The listing builds one solid part. Answer for the finished solid, in the listing's coordinates (mm). Face numbers are marked on the shaded views. A direction names the side the tool comes from. Coordinates: 2 decimals unless noted, no trailing zeros. Order: outer loops, then holes, each group sorted by start corner. A loop starts at its lowest first (then second) coordinate and runs counter-clockwise, first axis right, second up. Notation, with made-up numbers: (9.25, 53) -> (40.25, 53) arc R26 cw to (40.25, 85) -> close; hole circle Ø11 at (85, -34.5). An arc over 180 degrees is marked (long way). Return JSON: item names as keys, results as strings.
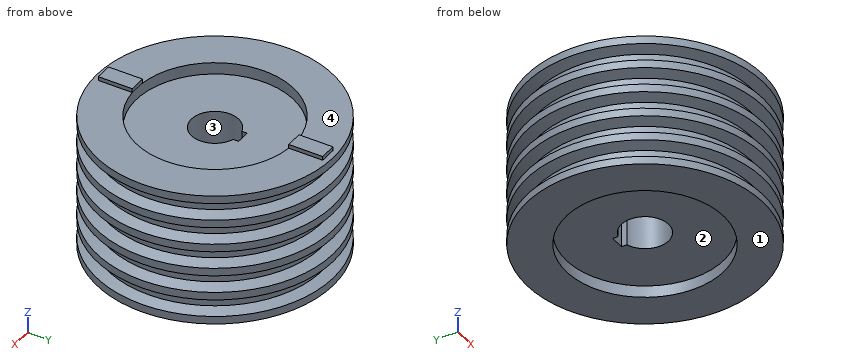
```python
from build123d import *

# Parameters (mm, degrees)
SKETCH1_R           = 150
BOSS_EXTRUDE1_DEPTH = 85
SKETCH3_R           = 30
CUT_EXTRUDE1_DEPTH  = 272.845544381
SKETCH4_R           = 100
SKETCH4_R_2         = 30
CUT_EXTRUDE2_DEPTH  = 15
SKETCH5_W           = 18
SKETCH5_H           = 11
CUT_EXTRUDE3_DEPTH  = 263.726093108
SKETCH10_W          = 21.256971554
SKETCH10_H          = 43.218095202
BOSS_EXTRUDE2_DEPTH = 5


with BuildPart() as part:
    # Sketch1 → Boss-Extrude1 (new, symmetric)
    with BuildSketch(Plane.XY):
        Circle(SKETCH1_R)
    extrude(amount=BOSS_EXTRUDE1_DEPTH, both=True)

    # Sketch3 → Cut-Extrude1 (cut, through all)
    with BuildSketch(Plane.XY.offset(85)):
        Circle(SKETCH3_R)
    extrude(amount=-CUT_EXTRUDE1_DEPTH, mode=Mode.SUBTRACT)

    # Sketch4 → Cut-Extrude2 (cut)
    with BuildSketch(Plane.XY.offset(85)):
        Circle(SKETCH4_R)
        Circle(SKETCH4_R_2, mode=Mode.SUBTRACT)
    cut_extrude2 = extrude(amount=-CUT_EXTRUDE2_DEPTH, mode=Mode.SUBTRACT)

    # Mirror1: Cut-Extrude2 across plane
    add(cut_extrude2.mirror(Plane.XY), mode=Mode.SUBTRACT)

    # Sketch5 → Cut-Extrude3 (cut, through all)
    with BuildSketch(Plane.XY.offset(70)):
        with Locations((0, 30)):
            Rectangle(SKETCH5_W, SKETCH5_H)
    extrude(amount=-CUT_EXTRUDE3_DEPTH, mode=Mode.SUBTRACT)

    # Sketch9 → Cut-Revolve2 (revolve, cut)
    with BuildSketch(Plane(origin=(0, 0, 0), x_dir=(1, 0, 0), z_dir=(0, 1, 0))):
        Polygon((150, 75), (136, 70.71977046), (136, 57.28022954), (150, 53), align=None)
        Polygon((150, 43), (150, 21), (136, 25.28022954), (136, 38.71977046), align=None)
        Polygon((150, 11), (136, 6.71977046), (136, -6.71977046), (150, -11), align=None)
        Polygon((150, -21), (150, -43), (136, -38.71977046), (136, -25.28022954), align=None)
        Polygon((150, -53), (136, -57.28022954), (136, -70.71977046), (150, -75), align=None)
    revolve(axis=Axis((0, 0, 0), (0, 0, -1)), mode=Mode.SUBTRACT)

    # Sketch10 → Boss-Extrude2 (add)
    with BuildSketch(Plane.XY.offset(85)):
        with Locations((-1.274543696, 121.17060528)):
            Rectangle(SKETCH10_W, SKETCH10_H)
        with Locations((-1.274543696, -121.17060528)):
            Rectangle(SKETCH10_W, SKETCH10_H)
    extrude(amount=BOSS_EXTRUDE2_DEPTH)


solid = part.part
```
Item 1: Flat-ended cylindrical pins translate along their axes: pin 1 (4 mm diameter, centred on y = 118, z = 87.5, fed in from +X); pin 2 (5 mm diameter, centred on x = -54, y = 117.5, fed in from +Z); pin 3 (5.5 mm diameter, centred on y = -129.5, z = 88.5, fed in from -X). Find the tip coordinate at first contact, or state that the pin passes through.
Answer list:
{"pin 1": "x = 9.35", "pin 2": "z = 85", "pin 3": "x = -11.9"}
Item 2: The part is cut by section A-A on z = 63. Determine the outline of the cut face in (x, y), plus the area to 3 significant figures.
Answer list:
{"outline": "circle Ø272 at (0, 0); hole (-9, 28.62) arc R30 ccw (long way) to (9, 28.62) -> (9, 35.5) -> (-9, 35.5) -> close", "area": "55,200 mm2"}
Item 3: Which of the six approach directions +Z, -Z, +X, -X, +Y, -Y give full straight-line access (tool end or side, diameter ignored) to the marked faces 1 and 2?
Answer list:
{"face 1": "-Z, +X, -X, +Y, -Y", "face 2": "-Z"}
Item 4: Find the intervals of material crossed by probe 1 along X at (y, z) = (0, 78); probe 2 along Z at (x, y) = (-80.5, -111.5), in increasing order.
Answer list:
{"probe 1": "-150 to -100, 100 to 150", "probe 2": "-85 to -71.19, -56.81 to -39.19, -24.81 to -7.19, 7.19 to 24.81, 39.19 to 56.81, 71.19 to 85"}
Item 5: Determine the mould class of the marked faces 3 and 4 for opening direction X: pulls with the +X half, pulls with the -X half, needs draft (parallel to the pull), parting line crosses it, or undercut.
Answer list:
{"face 3": "undercut", "face 4": "needs draft"}
